```python
from build123d import *

# Parameters (mm, degrees)
SKETCH_1_R          = 6
SKETCH_1_R_2        = 3
EXTRUDE_1_DEPTH     = 2
SKETCH_2_R          = 5
SKETCH_2_R_2        = 4
CUT_EXTRUDE_1_DEPTH = 0.5


with BuildPart() as part:
    # 草图1 → 凸台-拉伸1 (new, symmetric)
    with BuildSketch(Plane(origin=(0, 0, 0), x_dir=(1, 0, 0), z_dir=(0, 1, 0))):
        with Locations(Location((0, 0, 0), (0, 0, 270))):
            Circle(SKETCH_1_R)
        with Locations(Location((0, 0, 0), (0, 0, 270))):
            Circle(SKETCH_1_R_2, mode=Mode.SUBTRACT)
    extrude(amount=EXTRUDE_1_DEPTH, both=True)

    # 草图2 → 切除-拉伸1 (cut)
    with BuildSketch(Plane(origin=(0, 2, 0), x_dir=(1, 0, 0), z_dir=(0, 1, 0))):
        with Locations(Location((0, 0, 0), (0, 0, 270))):
            Circle(SKETCH_2_R)
        with Locations(Location((0, 0, 0), (0, 0, 270))):
            Circle(SKETCH_2_R_2, mode=Mode.SUBTRACT)
    cut_extrude_1 = extrude(amount=-CUT_EXTRUDE_1_DEPTH, mode=Mode.SUBTRACT)

    # 镜向1: 切除-拉伸1 across plane
    add(cut_extrude_1.mirror(Plane.ZX), mode=Mode.SUBTRACT)


solid = part.part
```
Can you work these out from the model? Positions are in its coordinate system, mm. A direction names the side the tool comes from. Coordinates: 2 decimals unless noted, no trailing zeros. Loops run counter-clockwise (first coordinate to the right, second up) from the corner with the lowest first, then second, coordinate; pieces in that order, holes last.
Item 1: Suppose I cut it at C-C (y = 0.8). Please give me the cut outline in (x, z), then the cut area to 3 significant figures.
Answers below:
outline: circle Ø12 at (0, 0); hole circle Ø6 at (0, 0)
area: 84.8 mm2
Item 2: Suppose I cut it at D-D (z = -3.5). Please give me the cut outline in (x, y).
Answers below:
outline: (-4.87, -2) - (-3.57, -2) - (-3.57, -1.5) - (-1.94, -1.5) - (-1.94, -2) - (1.94, -2) - (1.94, -1.5) - (3.57, -1.5) - (3.57, -2) - (4.87, -2) - (4.87, 2) - (3.57, 2) - (3.57, 1.5) - (1.94, 1.5) - (1.94, 2) - (-1.94, 2) - (-1.94, 1.5) - (-3.57, 1.5) - (-3.57, 2) - (-4.87, 2) - close
Item 3: If we mould it in two halves opening along X, with no side actions, what happens to faces 4 (the face through (1.802, 0.028, 5.723)), 5 (the face through (4, 2, -4)), 6 (the face through (-3.905, -1.754, -0.867))? For each: released by +X, released by -X, zero draft, split by the parting line, or undercut.
Answers below:
face 4: split by the parting line
face 5: zero draft
face 6: undercut
Item 4: Suppose I cut it at A-A (x = 0). Please give me the cut outline in (y, z).
Answers below:
outline: (-2, -6) - (2, -6) - (2, -5) - (1.5, -5) - (1.5, -4) - (2, -4) - (2, -3) - (-2, -3) - (-2, -4) - (-1.5, -4) - (-1.5, -5) - (-2, -5) - close; (-2, 3) - (2, 3) - (2, 4) - (1.5, 4) - (1.5, 5) - (2, 5) - (2, 6) - (-2, 6) - (-2, 5) - (-1.5, 5) - (-1.5, 4) - (-2, 4) - close
Item 5: Which directions (+Z, -Z, +X, -X, +Y, -Y) give clear straight access to the entire face, cutting with the end or side of a thin tool? Please do faces 1 (the face through (-4.88, 1.75, -1.08)), 2 (the face through (3, 2, 1)), 3 (the face through (-4.88, -1.75, -1.08)).
Answers below:
face 1: +Y
face 2: +Z, -Z, +X, -X, +Y
face 3: -Y
Item 6: I'm going to push flat-ended pins straight in: pin 1 (2 mm diameter, centred on y = 0, z = -2.5, fed in from -X); pin 2 (2 mm diameter, centred on y = 0, z = 3, fed in from +X). Where does each tip first touch, or does it pass through?
Answers below:
pin 1: stops at x = -5.81
pin 2: stops at x = 5.66
Item 7: Suppose I cut it at B-B (z = 0). Please give me the cut outline in (x, y).
Answers below:
outline: (-6, -2) - (-5, -2) - (-5, -1.5) - (-4, -1.5) - (-4, -2) - (-3, -2) - (-3, 2) - (-4, 2) - (-4, 1.5) - (-5, 1.5) - (-5, 2) - (-6, 2) - close; (3, -2) - (4, -2) - (4, -1.5) - (5, -1.5) - (5, -2) - (6, -2) - (6, 2) - (5, 2) - (5, 1.5) - (4, 1.5) - (4, 2) - (3, 2) - close
Item 8: Please list where these lines run through material, in increasing order: L1, parallel to X at y = -1.7, z = 0; L2, parallel to X at y = 1.15, z = 0; L3, parallel to Y at x = 4.5, z = 2.
Answers below:
L1: x = -6 to -5, -4 to -3, 3 to 4, 5 to 6
L2: x = -6 to -3, 3 to 6
L3: y = -1.5 to 1.5
